Autodesk Inventor part; units mm, degrees
ref_plane "YZ Plane" through (0, 0, 0) normal (1, 0, 0) x (0, 1, 0)
ref_plane "XZ Plane" through (0, 0, 0) normal (0, 1, 0) x (-1, 0, 0)
ref_plane "XY Plane" through (0, 0, 0) normal (0, 0, 1) x (1, 0, 0)
sketch "Sketch1" plane through (0, 0, 0) normal (0, 1, 0) x (-1, 0, 0)
  line L0 (-12.7, -31.75) -> (12.7, -31.75)
  line L1 (12.7, -31.75) -> (12.7, 31.75)
  line L2 (12.7, 31.75) -> (-12.7, 31.75)
  line L3 (-12.7, 31.75) -> (-12.7, -31.75)
  line L4 (-12.7, -31.75) -> (12.7, 31.75) construction
  line L5 (12.7, -31.75) -> (-12.7, 31.75) construction
  line L6 (-12.7, 19.05) -> (-44.323, 19.05)
  line L7 (-44.323, 19.05) -> (-44.323, -19.05)
  line L8 (-44.323, -19.05) -> (-12.7, -19.05)
  point P0 (0, 0)
  dimension "d0" = 25.4
  dimension "d1" = 63.5
  dimension "d21" = 31.623
  dimension "d22" = 12.7
  dimension "d23" = 12.7
extrude "Extrusion1" add sketch "Sketch1" along normal blind 3.175
sketch "Sketch2" plane through (0, 3.175, 0) normal (0, 1, 0) x (1, 0, 0)
  line L0 (0, -25.4) -> (0, 25.4) construction
  line L1 (-12.7, 31.75) -> (-12.7, -31.75) construction
  point P0 (0, 0)
  point P1 (0, 0)
  dimension "d4" = 50.8
hole "Hole1" at (0, 3.175, 25.4) at (0, 3.175, -25.4) direction (0, -1, 0) diameter 6.7564 end through all
sketch "Sketch3" plane through (0, 3.175, 0) normal (0, 1, 0) x (1, 0, 0)
  line L0 (44.323, -19.05) -> (44.323, 19.05) construction
  point P0 (0, 0)
  point P1 (18.9813, 0)
  point P2 (37.8968, 0)
  point P3 (0, 0)
  dimension "d13" = 18.9155
  dimension "d24" = 6.4262
hole "Hole2" at (18.9813, 3.175, 0) at (37.8968, 3.175, 0) direction (0, -1, 0) diameter 3.81 end through all
fillet "Fillet1" radius 3.175 8 edges at (12.7, 1.5875, 19.05) (12.7, 1.5875, 31.75) (-12.7, 1.5875, 31.75) (-12.7, 1.5875, -31.75) (12.7, 1.5875, -31.75) (12.7, 1.5875, -19.05) (44.323, 1.5875, -19.05) (44.323, 1.5875, 19.05)
properties part number "DB1-010" material "Polycarbonate, Smoke"
Part model, mm, in its own coordinate system. A direction names the side the tool comes from. Give positions to 0.01 mm unless a question says otherwise; leave off trailing zeros. Write each loop counter-clockwise with the first axis right and the second up, starting at its lowest first coordinate (ties: lowest second). Pieces come first, ordered by that corner, then holes.
1) Two-plate mould, pull along X, no slides. Class faces 3 (the face through (-11.75, 1.61, -30.84)), 4 (the face through (-0.149, 1.565, 22.025)), 5 (the face through (12.7, 2, -25)): released by +X, released by -X, zero draft, split by the parting line, or undercut.
Resolved:
face 3: released by -X
face 4: undercut
face 5: released by +X
2) Cut at B-B on x = 0. Write the cut outline in (y, z) (3 decimals).
Resolved:
outline: (0, -31.75) - (3.175, -31.75) - (3.175, -28.778) - (0, -28.778) - close; (0, -22.022) - (3.175, -22.022) - (3.175, 22.022) - (0, 22.022) - close; (0, 28.778) - (3.175, 28.778) - (3.175, 31.75) - (0, 31.75) - close
3) Cut at C-C on z = -25.4. Write the cut outline in (x, y) (3 decimals), then the cut area to 3 significant figures.
Resolved:
outline: (-12.7, 0) - (-3.378, 0) - (-3.378, 3.175) - (-12.7, 3.175) - close; (3.378, 0) - (12.7, 0) - (12.7, 3.175) - (3.378, 3.175) - close
area: 59.2 mm2
4) Pin check, flat tips, straight feed: pin 1 (6 mm diameter, centred on x = 0, z = -25.4, fed in from -Y); pin 2 (1.6 mm diameter, centred on y = 2, z = -26.5, fed in from +X); pin 3 (1 mm diameter, centred on x = 17.5, y = 2, fed in from -Z). Stop position of each tip, or through.
Resolved:
pin 1: passes through
pin 2: stops at x = 12.7
pin 3: stops at z = -19.05
5) Which spindle directions (+Z, -Z, +X, -X, +Y, -Y) get a long thin tool onto all of the face, cutting with end or side? Do faces 1 (the face through (12.7, 2, 25)), 2 (the face through (10, 0, 0)). Say none if no direction does.
Resolved:
face 1: +Z, +X, +Y, -Y
face 2: +Z, -Z, +X, -X, -Y
6) Probe L1, parallel to X at y = 1.3, z = 0; L2, parallel to Z at x = 0, y = 0.9; L3, parallel to X at y = 0.75, z = 25.4. List the from-to ranges inside material, lowest first.
Resolved:
L1: x = -12.7 to 17.08, 20.89 to 35.99, 39.8 to 44.32
L2: z = -31.75 to -28.78, -22.02 to 22.02, 28.78 to 31.75
L3: x = -12.7 to -3.38, 3.38 to 12.7
7) Cut at D-D on y = 1.55. Write the cut outline in (x, z) (3 decimals).
Resolved:
outline: (-12.7, -28.575) arc R3.175 ccw to (-9.525, -31.75) - (9.525, -31.75) arc R3.175 ccw to (12.7, -28.575) - (12.7, -22.225) arc R3.175 cw to (15.875, -19.05) - (41.148, -19.05) arc R3.175 ccw to (44.323, -15.875) - (44.323, 15.875) arc R3.175 ccw to (41.148, 19.05) - (15.875, 19.05) arc R3.175 cw to (12.7, 22.225) - (12.7, 28.575) arc R3.175 ccw to (9.525, 31.75) - (-9.525, 31.75) arc R3.175 ccw to (-12.7, 28.575) - close; hole circle Ø6.756 at (0, -25.4); hole circle Ø6.756 at (0, 25.4); hole circle Ø3.81 at (18.981, 0); hole circle Ø3.81 at (37.897, 0)
8) Cut at A-A on z = 0. Write the cut outline in (x, y) (3 decimals), then the cut area to 3 significant figures.
Resolved:
outline: (-12.7, 0) - (17.076, 0) - (17.076, 3.175) - (-12.7, 3.175) - close; (20.886, 0) - (35.992, 0) - (35.992, 3.175) - (20.886, 3.175) - close; (39.802, 0) - (44.323, 0) - (44.323, 3.175) - (39.802, 3.175) - close
area: 157 mm2
